Solid Edge part; units mm, degrees
sketch "Sketch1" plane through (0, 0, 0) normal (0, 0, 1) x (1, 0, 0)
  circle A0 centre (-87.4064, -37.8835) radius 5
  circle A1 centre (-87.4064, -37.8835) radius 10
  arc A2 (69.5936, 42.1165) -> (79.5936, 42.1165) centre (74.5936, 42.1165) cw
  line L0 (79.5936, 42.1165) -> (79.5936, 37.1165)
  arc A3 (79.5936, 37.1165) -> (69.5936, 37.1165) centre (74.5936, 37.1165) cw
  line L1 (69.5936, 37.1165) -> (69.5936, 42.1165)
  line L2 (84.5936, 42.1165) -> (84.5936, 37.1165)
  arc A4 (64.5936, 42.1165) -> (84.5936, 42.1165) centre (74.5936, 42.1165) cw
  line L3 (64.5936, 37.1165) -> (64.5936, 42.1165)
  arc A5 (84.5936, 37.1165) -> (64.5936, 37.1165) centre (74.5936, 37.1165) cw
  circle A6 centre (74.5936, -37.8835) radius 5
  circle A7 centre (74.5936, -37.8835) radius 10
  line L4 (-77.4064, 42.1165) -> (-77.4064, 37.1165)
  arc A8 (-77.4064, 37.1165) -> (-97.4064, 37.1165) centre (-87.4064, 37.1165) cw
  line L5 (-97.4064, 37.1165) -> (-97.4064, 42.1165)
  arc A9 (-97.4064, 42.1165) -> (-77.4064, 42.1165) centre (-87.4064, 42.1165) cw
  line L6 (-92.4064, 37.1165) -> (-92.4064, 42.1165)
  arc A10 (-82.4064, 37.1165) -> (-92.4064, 37.1165) centre (-87.4064, 37.1165) cw
  line L7 (-82.4064, 42.1165) -> (-82.4064, 37.1165)
  arc A11 (-92.4064, 42.1165) -> (-82.4064, 42.1165) centre (-87.4064, 42.1165) cw
extrude "Protrusion1" add sketch "Sketch1" against normal blind 2
sketch "Sketch2" plane through (-87.4064, -37.8835, 0) normal (0, 0, 1) x (1, 0, 0)
  arc A0 (5, 75) -> (-5, 75) centre (0, 75) cw
  line L0 (-5, 75) -> (-5, 80)
  arc A1 (-5, 80) -> (5, 80) centre (0, 80) cw
  line L1 (5, 80) -> (5, 75)
  circle A2 centre (0, 0) radius 5
  circle A3 centre (162, 0) radius 5
  arc A4 (167, 75) -> (157, 75) centre (162, 75) cw
  line L2 (157, 75) -> (157, 80)
  arc A5 (157, 80) -> (167, 80) centre (162, 80) cw
  line L3 (167, 80) -> (167, 75)
  line L4 (30, -25) -> (137, -25)
  line L5 (137, -25) -> (137, -20)
  line L6 (137, -20) -> (167.4546, -9.5523)
  arc A6 (173, 0) -> (167.4546, -9.5523) centre (162, 0) cw
  line L7 (173, 80) -> (173, 0)
  arc A7 (162, 91) -> (173, 80) centre (162, 80) cw
  line L8 (0, 91) -> (162, 91)
  arc A8 (-11, 80) -> (0, 91) centre (0, 80) cw
  line L9 (-11, 80) -> (-11, 0)
  arc A9 (-11, 0) -> (-5.4546, -9.5523) centre (0, 0) ccw
  line L10 (-5.4546, -9.5523) -> (30, -20)
  line L11 (30, -20) -> (30, -25)
  dimension "D1" = 30
extrude "ExtrudedProtrusion_2" add sketch "Sketch2" along normal blind 10
sketch "Sketch3" plane through (-6.4064, 53.1165, 5) normal (0, 1, 0) x (-1, 0, 0)
  arc A0 (41, 15) -> (51, 5) centre (51, 15) ccw
  line L0 (-46, 15) -> (41, 15)
  arc A1 (-56, 5) -> (-46, 15) centre (-56, 15) ccw
  line L1 (-56, 5) -> (51, 5)
extrude "Protrusion2" add sketch "Sketch3" along normal up to surface (116 mm away) from surface at -116
fillet "Round_1" radius 5 2 edges at (-57.4064, -62.8835, 5) (49.5936, -62.8835, 5)
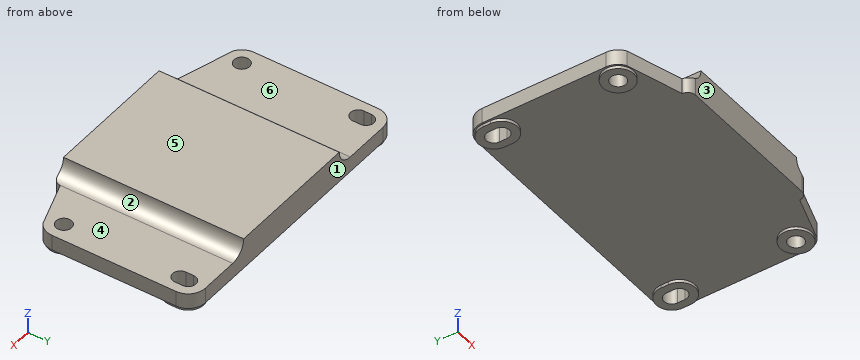
Check sheet for the modelled part. Datum: model origin and axes. Units: mm. Face numbers are marked on the shaded views. A direction names the side the tool comes from. Give positions to 0.01 mm unless a question says otherwise; leave off trailing zeros. Write each loop counter-clockwise with the first axis right and the second up, starting at its lowest first coordinate (ties: lowest second). Pieces come first, ordered by that corner, then holes. Notation, with made-up numbers: (-23, 14) -> (-19, 14) arc R30 ccw to (-19, 50) -> close; hole circle Ø9 at (12, 75). An arc over 180 degrees is marked (long way). Write item = value, one per line.
Item 1: Sectioned sample at D-D on x = -24. Record the boundary of the cut face in (y, z).
Output:
outline = (-62.88, 0) -> (53.12, 0) -> (53.12, 20) -> (-62.88, 20) -> close
Item 2: Tool access check on the marked faces 4, 5 and 6. Record the directions out of +Z, -Z, +X, -X, +Y, -Y that give a thin tool (end or side, any length) a straight path to the whole face; none if there is none.
Output:
face_4 = +Z, +X, +Y, -Y
face_5 = +Z, +X, -X, +Y, -Y
face_6 = +Z, -X, +Y, -Y
Item 3: Sectioned sample at A-A on z = 2.25. Count the separate pieces of the cut face and the enclosed holes in it, and give its area (3 significant figures).
Output:
separate_pieces = 1
enclosed_holes = 4
area = 20,000 mm^2
Item 4: Scan lines: probe 1 along Y at (x, z) = (78, 0.75); probe 2 along Y at (x, z) = (74.5, 2.25); probe 3 along Z at (x, y) = (-82, 6). Record each from-to range of solid material in increasing order. Write a range as from..to.
Output:
probe_1 = -48.14..-41.54, -34.22..33.46, 45.78..52.58
probe_2 = -49.34..-42.88, -32.88..32.12, 47.12..53.12
probe_3 = 0..10
Item 5: Gauge pin test, flat ends, axial feed: pin 1 (3 mm diameter, centred on x = -78, y = 8.5, fed in from +Z); pin 2 (0.6 mm diameter, centred on y = 40.5, z = -1.5, fed in from +X); pin 3 (12 mm diameter, centred on x = -40.5, y = -17, fed in from -Z). Record the tip position at first contact, or that the pin passes through.
Output:
pin_1 = 10
pin_2 = 84.59
pin_3 = 0
Item 6: Release check for a two-part mould opening along Y. For the marked faces 1, 2 and 3 record: +Y half, -Y half, draft (parallel to the pull), parting line (faces both ways), or undercut.
Output:
face_1 = +Y half
face_2 = draft
face_3 = -Y half
Item 7: Sectioned sample at C-C on y = -36. Record the boundary of the cut face in (x, z), and give its area (3 significant figures).
Output:
outline = (-98.41, 0) -> (-97.23, 0) -> (-97.23, -2) -> (-92.04, -2) -> (-92.04, 10) -> (-98.41, 10) -> close; (-82.77, -2) -> (-77.59, -2) -> (-77.59, 0) -> (64.77, 0) -> (64.77, -2) -> (69.96, -2) -> (69.96, 10) -> (49.59, 10) arc R10 cw to (39.59, 20) -> (-47.41, 20) arc R10 cw to (-57.41, 10) -> (-82.77, 10) -> close; (79.23, -2) -> (84.41, -2) -> (84.41, 0) -> (85.59, 0) -> (85.59, 10) -> (79.23, 10) -> close
area = 2,610 mm^2
Item 8: Sectioned sample at B-B on y = -13. Record the boundary of the cut face in (x, z).
Output:
outline = (-98.41, 0) -> (85.59, 0) -> (85.59, 10) -> (49.59, 10) arc R10 cw to (39.59, 20) -> (-47.41, 20) arc R10 cw to (-57.41, 10) -> (-98.41, 10) -> close
